Read the model definition and answer for the solid it produces. Units are mm, in the model's axes. A direction names the side the tool comes from. Give positions to 0.01 mm unless a question says otherwise; leave off trailing zeros. Order: outer loops, then holes, each group sorted by start corner. A loop starts at its lowest first (then second) coordinate and runs counter-clockwise, first axis right, second up. Notation, with made-up numbers: (30, 71) - (41, 71) arc R27 cw to (41, 105) - close; hole circle Ø4 at (59.25, -37.5). An arc over 180 degrees is marked (long way). Return JSON: item names as keys, results as strings.
```python
from build123d import *

# Parameters (mm, degrees)
ESBO_O1_W                = 90
ESBO_O1_H                = 70
RESSALTO_EXTRUS_O1_DEPTH = 1.5
ESBO_O2_R                = 2
CORTE_EXTRUS_O1_DEPTH    = 1.5
ESBO_O3_R                = 11
RESSALTO_EXTRUS_O2_DEPTH = 44


with BuildPart() as part:
    # Esboço1 → Ressalto-extrusão1 (new body)
    with BuildSketch(Plane(origin=(0, 0, 0), x_dir=(1, 0, 0), z_dir=(0, 1, 0))):
        with Locations((45, 35)):
            Rectangle(ESBO_O1_W, ESBO_O1_H)
    extrude(amount=RESSALTO_EXTRUS_O1_DEPTH)

    # Esboço2 → Corte-extrusão1 (cut)
    with BuildSketch(Plane(origin=(0, 1.5, 0), x_dir=(1, 0, 0), z_dir=(0, 1, 0))):
        with Locations((87, 3)):
            Circle(ESBO_O2_R)
        with Locations((87, 67)):
            Circle(ESBO_O2_R)
        with Locations((3, 3)):
            Circle(ESBO_O2_R)
        with Locations((3, 67)):
            Circle(ESBO_O2_R)
    extrude(amount=-CORTE_EXTRUS_O1_DEPTH, mode=Mode.SUBTRACT)

    # Esboço3 → Ressalto-extrusão2 (add)
    with BuildSketch(Plane(origin=(0, 1.5, 0), x_dir=(1, 0, 0), z_dir=(0, 1, 0))):
        with Locations((71, 25)):
            Circle(ESBO_O3_R)
        Polygon((15, 0), (15, -6), (57, -6), (57, 0), (57, 18), (15, 18), align=None)
    extrude(amount=RESSALTO_EXTRUS_O2_DEPTH)


solid = part.part
```
Q1. A cutting plane is placed at D-D (z = -25). Write down the section's boundary in (x, y).
Values:
{"outline": "(0, 0) - (90, 0) - (90, 1.5) - (82, 1.5) - (82, 45.5) - (60, 45.5) - (60, 1.5) - (0, 1.5) - close"}
Q2. A cutting plane is placed at B-B (y = 4). Write down the section's boundary in (x, z), and give its area (3 significant figures).
Values:
{"outline": "(15, -18) - (57, -18) - (57, 6) - (15, 6) - close; circle Ø22 at (71, -25)", "area": "1,390 mm²"}
Q3. Determine the mould class of faces 4 (the cylindrical face through (3, 1, -1)), 5 (the flat face through (15, 23, -6)), 6 (the flat face through (36, 23, -18)) for opening direction Z: released by +Z, released by -Z, zero draft, split by the parting line, or undercut.
Values:
{"face 4": "undercut", "face 5": "zero draft", "face 6": "released by -Z"}
Q4. A cutting plane is placed at A-A (z = -67). Write down the section's boundary in (x, y).
Values:
{"outline": "(0, 0) - (1, 0) - (1, 1.5) - (0, 1.5) - close; (5, 0) - (85, 0) - (85, 1.5) - (5, 1.5) - close; (89, 0) - (90, 0) - (90, 1.5) - (89, 1.5) - close"}
Q5. A cutting plane is placed at C-C (x = 3). Write down the section's boundary in (y, z), and give its area (3 significant figures).
Values:
{"outline": "(0, -70) - (1.5, -70) - (1.5, -69) - (0, -69) - close; (0, -65) - (1.5, -65) - (1.5, -5) - (0, -5) - close; (0, -1) - (1.5, -1) - (1.5, 0) - (0, 0) - close", "area": "93.0 mm²"}
Q6. Given pin 1 (6.5 mm diameter, centred on x = 35, z = 4.5, fed in from -Y); pin 2 (19 mm diameter, centred on y = 30, z = -9, fed in from -X); pin 3 (8 mm diameter, centred on y = 14.5, z = -19, fed in from +X), each flat-ended and moving along its own axis, determine where each tip first touches the part or whether it passes through.
Values:
{"pin 1": "stops at y = 1.5", "pin 2": "stops at x = 15", "pin 3": "stops at x = 81.82"}
Q7. Consider L1, parallel to X at y = 1.1, z = -67; L2, parallel to Z at x = 3, y = 0.4; L3, parallel to Y at x = 44, z = -41. Determine where each line is inside the solid, lowest interval first.
Values:
{"L1": "x = 0 to 1, 5 to 85, 89 to 90", "L2": "z = -70 to -69, -65 to -5, -1 to 0", "L3": "y = 0 to 1.5"}
Q8. For faces 1 (the flat face through (44, 0, -35)), 2 (the cylindrical face through (62.27, 23.19, -18.31)), 3 (the flat face through (36, 1.5, 3)), determine the directions among +Z, -Z, +X, -X, +Y, -Y from which every point of the face is accessible in a straight line to the end or side of a thin tool.
Values:
{"face 1": "+Z, -Z, +X, -X, -Y", "face 2": "+Y", "face 3": "+Z, +X, -X, -Y"}
